```python
from build123d import *

# Parameters (mm, degrees)
BOSS_EXTRUDE1_DEPTH           = 4
DRAFT1_ANGLE                  = 45.000000004
DRAFT2_ANGLE                  = 45.000000005
F_4_0_4_DIAMETER_HOLE1_D      = 4
CSK_FOR_M3_SFHCS1_D           = 2.5
CSK_FOR_M3_SFHCS1_CSINK_D     = 4
CSK_FOR_M3_SFHCS1_CSINK_ANGLE = 90
FILLET1_R                     = 1
FILLET2_R                     = 6.5
HOLE2_D                       = 10
HOLE2_CBORE_D                 = 12
HOLE2_CBORE_DEPTH             = 1


with BuildPart() as part:
    # Sketch1 → Boss-Extrude1 (new body)
    with BuildSketch(Plane.XZ.offset(2)):
        with BuildLine():
            Line((11.12, 26.5), (-6.5, 26.5))
            Line((-6.5, 26.5), (-6.5, 0))
            ThreePointArc((-6.5, 0), (3e-09, -6.500000003), (6.500000005, 0))
            Line((6.500000005, 0), (6.500000005, 20.5))
            Line((6.500000005, 20.5), (13.605281374, 20.5))
            Line((13.605281374, 20.5), (13.605281374, 36.100603473))
            Line((13.605281374, 36.100603473), (11.12, 38.585884847))
            Line((11.12, 38.585884847), (11.12, 26.5))
        make_face()
    extrude(amount=-BOSS_EXTRUDE1_DEPTH)

    # Draft1
    draft1_faces = [part.faces().sort_by_distance(p)[0] for p in [
        (13.605281374, 0, 28.300301737),
    ]]
    draft(draft1_faces, Plane(origin=(6.500000005, 2, 20.5), x_dir=(-1, 0, 0), z_dir=(0, 0, -1)), DRAFT1_ANGLE)

    # Draft2
    draft2_faces = [part.faces().sort_by_distance(p)[0] for p in [
        (11.12, 0, 32.542942424),
    ]]
    draft(draft2_faces, Plane(origin=(11.12, 2, 26.5), x_dir=(1, 0, 0), z_dir=(0, 0, 1)), DRAFT2_ANGLE)

    # Ø4.0 (4) Diameter Hole1 (through all)
    with Locations(Plane(origin=(0, 2, 0), x_dir=(1, 0, 0), z_dir=(0, 1, 0))):
        with Locations((0, 2.5)):
            Hole(F_4_0_4_DIAMETER_HOLE1_D / 2)

    # CSK for M3 SFHCS1 (through all)
    with Locations(Plane(origin=(0, -2, 0), x_dir=(-1, 0, 0), z_dir=(0, -1, 0))):
        with Locations((-14.690228422, -24.413374173), (-18.225762328, -27.948908079)):
            CounterSinkHole(CSK_FOR_M3_SFHCS1_D / 2, CSK_FOR_M3_SFHCS1_CSINK_D / 2, counter_sink_angle=CSK_FOR_M3_SFHCS1_CSINK_ANGLE)

    # Fillet1
    fillet1_edges = [part.edges().sort_by_distance(p)[0] for p in [
        (13.605281374, 0, 20.5),
        (6.500000005, 0, 20.5),
        (11.12, 0, 26.5),
    ]]
    fillet(fillet1_edges, radius=FILLET1_R)

    # Fillet2
    fillet2_edges = [part.edges().sort_by_distance(p)[0] for p in [
        (-6.5, 0, 26.5),
    ]]
    fillet(fillet2_edges, radius=FILLET2_R)

    # Hole2 (through all)
    with Locations(Plane(origin=(0, 2, 20), x_dir=(0, 0, 1), z_dir=(0, 1, 0))):
        with Locations((0, 0)):
            CounterBoreHole(HOLE2_D / 2, HOLE2_CBORE_D / 2, HOLE2_CBORE_DEPTH)


solid = part.part
```
Read the model definition and answer for the solid it produces. Units are mm, in the model's axes. A direction names the side the tool comes from. Give positions to 0.01 mm unless a question says otherwise; leave off trailing zeros. Write each loop counter-clockwise with the first axis right and the second up, starting at its lowest first coordinate (ties: lowest second). Pieces come first, ordered by that corner, then holes. Notation, with made-up numbers: (72, 19) -> (95, 19) arc R12 ccw to (95, 26) -> close; hole circle Ø2 at (74.25, 24.5). An arc over 180 degrees is marked (long way). Answer in a Markdown table with one row per item.
1) Section D-D on z = 22 is taken. Give the vertices of the cut face in (x, y).
Results list:
| item | result |
|---|---|
| outline | (-6.18, -2) -> (-4.58, -2) -> (-4.58, 1) -> (-5.66, 1) -> (-5.66, 2) -> (-6.18, 2) -> close; (4.58, -2) -> (15.11, -2) -> (15.11, 2) -> (5.66, 2) -> (5.66, 1) -> (4.58, 1) -> close |
2) This flat-tipped pin is pushed along its axis until it touches: pin 1 Ø11.5 at (x, z) = (0, 20) entering from +Y. Where does it stop, or does it pass through?
Results list:
| item | result |
|---|---|
| pin 1 | y = 1 |
3) Straight lines are drawn through the part: line 1 (Z direction, x = -0.5, y = -0.95); line 2 (Z direction, x = 0.5, y = 1.85); line 3 (X direction, y = -1.35, z = 17.5). For each, find the intervals that lie inside material, in ascending order. Write a range as [from, to].
Results list:
| item | result |
|---|---|
| line 1 | [-6.48, -4.44], [-0.56, 15.03], [24.97, 26.48] |
| line 2 | [-6.48, -4.44], [-0.56, 14.02], [25.98, 26.5] |
| line 3 | [-6.5, -4.33], [4.33, 6.5] |
4) Section A-A on z = -2.5 is taken. Give the vertices of the cut face in (x, y).
Results list:
| item | result |
|---|---|
| outline | (-6, -2) -> (-2, -2) -> (-2, 2) -> (-6, 2) -> close; (2, -2) -> (6, -2) -> (6, 2) -> (2, 2) -> close |
5) Section C-C on z = 8 is taken. Give the vertices of the cut face in (x, y).
Results list:
| item | result |
|---|---|
| outline | (-6.5, -2) -> (6.5, -2) -> (6.5, 2) -> (-6.5, 2) -> close |
6) Section B-B on y = 0.4 is taken. Give the vertices of the cut face in (x, z), plus the area to 3 significant figures.
Results list:
| item | result |
|---|---|
| outline | (-6.5, 0) arc R6.5 ccw to (6.5, 0) -> (6.5, 19.5) arc R1 cw to (7.5, 20.5) -> (13.19, 20.5) arc R1 ccw to (13.9, 20.79) -> (21.41, 28.3) -> (17.16, 32.54) -> (11.41, 26.79) arc R1 cw to (10.71, 26.5) -> (0, 26.5) arc R6.5 ccw to (-6.5, 20) -> close; hole circle Ø10 at (0, 20); hole circle Ø4 at (0, -2.5); hole circle Ø2.5 at (14.69, 24.41); hole circle Ø2.5 at (18.23, 27.95) |
| area | 395 mm^2 |
7) Determine the mould class of faces 4 (the cylindrical face through (-2.3, 1.51, 25.54)), 5 (the flat face through (17.599, -0.028, 24.494)), 6 (the flat face through (5, 0, 26.5)) for opening direction X: released by +X, released by -X, zero draft, split by the parting line, or undercut.
Results list:
| item | result |
|---|---|
| face 4 | undercut |
| face 5 | released by +X |
| face 6 | zero draft |
8) A tool of negligible diameter and unlimited length cuts with its end or side. For faces 1 (the flat face through (6.5, 0, 10)), 2 (the cylindrical face through (-4.545, 0.028, 24.646)), 3 (the flat face through (4, 1, 16)), from which of +Z, -Z, +X, -X, +Y, -Y can it reach the whole face along a straight path? Write none if from no direction.
Results list:
| item | result |
|---|---|
| face 1 | -Z, +X, +Y, -Y |
| face 2 | +Z, -X, +Y, -Y |
| face 3 | +Y |
